```python
from build123d import *
from build123d import SkipClean  # not in build123d's __all__

# Parameters (mm, degrees)
F0_W          = 10.3
F0_H          = 5
F1_DEPTH      = 10
F3_DEPTH      = 10.3
F4_DEPTH      = 11
F5_W          = 4
F5_H          = 2
F6_DEPTH      = 2
F6_DEPTH_BACK = 5
F7_W          = 6.2
F7_H          = 3
F8_DEPTH      = 8.5
F10_W         = 6.2
F10_H         = 2
F11_DEPTH     = 25
F7_W_2        = 10.3
F7_H_2        = 5
F12_DEPTH     = 4


with BuildPart() as f1:
    # F0 (on Front) → F1 (new body)
    with BuildSketch(Plane.XZ):
        Rectangle(F0_W, F0_H)
    extrude(amount=F1_DEPTH)

    # F2 (on face) → F3 (join)
    with BuildSketch(Plane(origin=(-5.15, 0, 0), x_dir=(0, -1, 0), z_dir=(-1, 0, 0))):
        with BuildLine():
            ThreePointArc((0, -1.2), (-1.2, 0), (0, 1.2))
            Line((0, 1.2), (0, 2.5))
            Line((0, 2.5), (2.4494897428, 2.5))
            ThreePointArc((2.4494897428, 2.5), (-3.5, 0), (2.4494897428, -2.5))
            Line((2.4494897428, -2.5), (0, -2.5))
            Line((0, -2.5), (0, -1.2))
        make_face()
    extrude(amount=-F3_DEPTH)

    # F2 (on face) → F4 (cut)
    with BuildSketch(Plane(origin=(-5.15, 0, 0), x_dir=(0, -1, 0), z_dir=(-1, 0, 0))):
        with BuildLine():
            ThreePointArc((0, -1.2), (0.8485281374, -0.8485281374), (1.2, 0))
            ThreePointArc((1.2, 0), (0.8485281374, 0.8485281374), (0, 1.2))
            Line((0, 1.2), (0, -1.2))
        make_face()
    with SkipClean():  # cleaning this boolean's faces spoils the solid; the shape is the same uncleaned
        extrude(amount=-F4_DEPTH, mode=Mode.SUBTRACT)

    # F5 (on face) → F6 (cut, two sides)
    with BuildSketch(Plane.XY.offset(2.5)) as f6_sk:
        with Locations((0, -2.3844429548)):
            Rectangle(F5_W, F5_H)
    extrude(amount=-F6_DEPTH, mode=Mode.SUBTRACT)
    extrude(f6_sk.sketch, amount=F6_DEPTH_BACK, mode=Mode.SUBTRACT)

    # F7 (on face) → F8 (cut)
    with BuildSketch(Plane.XZ.offset(10)):
        Rectangle(F7_W, F7_H)
    extrude(amount=-F8_DEPTH, mode=Mode.SUBTRACT)

    # F10 (on face) → F11 (cut)
    with BuildSketch(Plane(origin=(0, -6.4174682453, -3.7051270189), x_dir=(1, 0, 0), z_dir=(0, -0.8660254038, -0.5))):
        with Locations((0, 3.5294059198)):
            Rectangle(F10_W, F10_H)
    extrude(amount=-F11_DEPTH, mode=Mode.SUBTRACT)

    # F7 (on face) → F12 (join)
    with BuildSketch(Plane.XZ.offset(10)):
        Rectangle(F7_W_2, F7_H_2)
        Rectangle(F7_W, F7_H, mode=Mode.SUBTRACT)
    extrude(amount=F12_DEPTH)


solid = f1.part
```
Geometry: final body of the model. Coordinates: model frame, mm. A direction names the side the tool comes from. Round coordinates to 2 decimals unless told otherwise and drop trailing zeros. Loops run counter-clockwise (first coordinate to the right, second up) from the corner with the lowest first, then second, coordinate; pieces in that order, holes last. Notation, with made-up numbers: (71, -8) -> (86, -8) arc R18 cw to (86, 21) -> close; hole circle Ø4 at (64, 55). An arc over 180 degrees is marked (long way). Use one line per item in the form item = value.
Item 1: Material intervals for probe 1 along X at (y, z) = (-7.25, 0.5); probe 2 along Z at (x, y) = (-2.25, -7); probe 3 along Y at (x, z) = (-0.5, 0), sorted ascending.
Evaluation:
probe_1 = -5.15 to -3.1, 3.1 to 5.15
probe_2 = -2.5 to -1.5, 1.5 to 2.5
probe_3 = -1.5 to -1.2, 1.2 to 3.5
Item 2: Cut plane A-A on x = -1.75. Give the number of separate pieces and of enclosed holes in the cut face, then the cut area to 3 significant figures.
Evaluation:
separate_pieces = 2
enclosed_holes = 1
area = 44.4 mm2
Item 3: Cut plane D-D on x = -4. Output: boundary loops of the cut face in (y, z), then the cut area to 3 significant figures.
Evaluation:
outline = (-14, -2.5) -> (-2.45, -2.5) arc R3.5 ccw (long way) to (-2.45, 2.5) -> (-14, 2.5) -> close; hole circle Ø2.4 at (0, 0)
area = 88.1 mm2
Item 4: Contact query for flat-ended pins moving along their axis: pin 1 Ø6 at (x, y) = (-2.5, -9.5) entering from +Z; pin 2 Ø0.8 at (x, y) = (-2.5, -2) entering from -Z; pin 3 Ø5 at (x, y) = (4, -8) entering from -Z; pin 4 Ø4 at (x, z) = (1, 1.5) entering from +Y. Output: stop coordinate, or through.
Evaluation:
pin_1 = 2.5
pin_2 = -3.11
pin_3 = -2.5
pin_4 = 3.5
Item 5: Cut plane C-C on y = -1. Output: boundary loops of the cut face in (x, z), then the cut area to 3 significant figures.
Evaluation:
outline = (-5.15, -3.35) -> (5.15, -3.35) -> (5.15, -0.66) -> (-5.15, -0.66) -> close; (-5.15, 0.66) -> (5.15, 0.66) -> (5.15, 3.35) -> (3.1, 3.35) -> (3.1, 2.34) -> (-3.1, 2.34) -> (-3.1, 3.35) -> (-5.15, 3.35) -> close
area = 49.2 mm2
Item 6: Draft query along Y for faces 1 (the cylindrical face through (-0.07, 3.09, -1.64)), 2 (the flat face through (-2.6, -2, 1.5)), 3 (the flat face through (-0.04, -0.47, 2.65)). Return one class per face: released by +Y, released by -Y, zero draft, split by the parting line, or undercut.
Evaluation:
face_1 = split by the parting line
face_2 = zero draft
face_3 = undercut
Item 7: Access query for faces 4 (the flat face through (2.5, -2, 1.5)), 5 (the flat face through (-0.04, -5.61, 1.99)), 6 (the flat face through (0, -8, 2.5)). Directions: +Z, -Z, +X, -X, +Y, -Y. A direction counts if a zero-diameter tool reaches every point of the face in a straight line with its end or side. Return the directions, or none.
Evaluation:
face_4 = -Y
face_5 = none
face_6 = +Z, +X, -X, -Y
Item 8: Cut plane B-B on z = 0.75. Output: boundary loops of the cut face in (x, y), then the cut area to 3 significant figures.
Evaluation:
outline = (-5.15, -14) -> (-3.1, -14) -> (-3.1, -1.5) -> (-2, -1.5) -> (-2, -1.38) -> (2, -1.38) -> (2, -1.5) -> (3.1, -1.5) -> (3.1, -14) -> (5.15, -14) -> (5.15, -0.94) -> (-5.15, -0.94) -> close; (-5.15, 0.94) -> (5.15, 0.94) -> (5.15, 3.42) -> (-5.15, 3.42) -> close
area = 82.2 mm2
